```python
from build123d import *

# Parameters (mm, degrees)
TD_SKETCH_R                             = 0.79248
TL_FEATURE_DEPTH                        = 21.0312
TDF_STD_SKETCH_W                        = 2.09296
TDF_STD_SKETCH_H                        = 2.09296
TDF_STD_FEATURE_DEPTH                   = 22.061040395
ISA_20_STD_FEATURE_DEPTH                = 22.061040395
ISA_20_STD_FEATURE_DEPTH_BACK           = 22.061040395
VW_STD_FEATURE_DEPTH                    = 22.061040395
VW_STD_FEATURE_DEPTH_BACK               = 22.061040395
F_10BA_STD_FEATURE_DEPTH                = 22.061040503
F_10BA_STD_FEATURE_DEPTH_BACK           = 22.061040503
FRO_STD_FEATURE_DEPTH                   = 22.061040395
FRO_STD_FEATURE_DEPTH_BACK              = 22.061040395
C_STD_FEATURE_DEPTH                     = 22.061040395
C_STD_FEATURE_DEPTH_BACK                = 22.061040395
ERW_STD_FEATURE_DEPTH                   = 0.018159984
H_STD_FEATURE_REACH                     = 22.957
H_STD_SKETCH_R                          = 0.01778
H_STD_SKETCH_3_R                        = 0.01778
FUNNEL_FINAL_DIAMETRE_STD_FEATURE_DEPTH = 2.499995
FUNNEL_FINAL_DIAMETRE_STD_FEATURE_DRAFT = -22.5
ROUND_BR_STD_FEATURE_START              = -1
ROUND_BR_STD_FEATURE_DEPTH              = 0.936596355


with BuildPart() as part:
    # TD_sketch → TL_feature (new body)
    with BuildSketch(Plane(origin=(0, 0, 0), x_dir=(1, 0, 0), z_dir=(0, 1, 0))):
        with Locations(Location((0, 0, 0), (0, 0, 270))):
            Circle(TD_SKETCH_R)
    extrude(amount=TL_FEATURE_DEPTH)

    # TDF_STD_sketch → TDF_STD_feature (cut, through all)
    with BuildSketch(Plane(origin=(0, 0, 0), x_dir=(1, 0, 0), z_dir=(0, 1, 0))):
        with Locations((-1.4224, 0)):
            Rectangle(TDF_STD_SKETCH_W, TDF_STD_SKETCH_H)
    extrude(amount=TDF_STD_FEATURE_DEPTH, mode=Mode.SUBTRACT)

    # ISA_20_STD_sketch → ISA_20_STD_feature (cut, two sides: drawn at the far end of the back side and taken through both)
    with BuildSketch(Plane(origin=(0, 0, 0), x_dir=(0, 0, -1), z_dir=(1, 0, 0)).offset(-ISA_20_STD_FEATURE_DEPTH_BACK)):
        Polygon((-12.948362797, 73.253751326), (-3.740117997, 21.0312), (-0.03175, 0), (0.03175, 0), (3.740117997, 21.0312), (12.948362797, 73.253751326), (12.948362797, -32.802585388), (-12.948362797, -32.802585388), align=None)
    extrude(amount=ISA_20_STD_FEATURE_DEPTH + ISA_20_STD_FEATURE_DEPTH_BACK, mode=Mode.SUBTRACT)

    # VW_STD_sketch → VW_STD_feature (cut, two sides: drawn at the far end of the back side and taken through both)
    with BuildSketch(Plane(origin=(0, 0, 0), x_dir=(0, 0, -1), z_dir=(1, 0, 0)).offset(-VW_STD_FEATURE_DEPTH_BACK)):
        with BuildLine():
            Line((-70.567982417, 70.76464549), (-20.834536927, 21.0312))
            Line((-20.834536927, 21.0312), (-0.060418463, 0.257081537))
            ThreePointArc((-0.060418463, 0.257081537), (-0.04390038, 0.232360478), (-0.0381, 0.2032))
            Line((-0.0381, 0.2032), (-0.0381, 0))
            Line((-0.0381, 0), (0.0381, 0))
            Line((0.0381, 0), (0.0381, 0.2032))
            ThreePointArc((0.0381, 0.2032), (0.04390038, 0.232360478), (0.060418463, 0.257081537))
            Line((0.060418463, 0.257081537), (20.834536927, 21.0312))
            Line((20.834536927, 21.0312), (70.567982417, 70.76464549))
            Line((70.567982417, 70.76464549), (70.567982417, -69.902780741))
            Line((70.567982417, -69.902780741), (-70.567982417, -69.902780741))
            Line((-70.567982417, -69.902780741), (-70.567982417, 70.76464549))
        make_face()
    extrude(amount=VW_STD_FEATURE_DEPTH + VW_STD_FEATURE_DEPTH_BACK, mode=Mode.SUBTRACT)

    # 10BA_STD_sketch → 10BA_STD_feature (cut, two sides: drawn at the far end of the back side and taken through both)
    with BuildSketch(Plane.XY.offset(-F_10BA_STD_FEATURE_DEPTH_BACK)):
        Polygon((-53.187772193, 0), (-0.37592, 0), (-0.2921, 0), (-0.091550146, 0.028185444), (3.611847997, 21.0312), (12.782529889, 73.04072149), (91.167207648, 2.243763782), (25.196905566, -70.796957708), align=None)
    extrude(amount=F_10BA_STD_FEATURE_DEPTH + F_10BA_STD_FEATURE_DEPTH_BACK, mode=Mode.SUBTRACT)

    # FRO_STD_sketch → FRO_STD_feature (cut, two sides: drawn at the far end of the back side and taken through both)
    with BuildSketch(Plane.XY.offset(-FRO_STD_FEATURE_DEPTH_BACK)):
        with BuildLine():
            Line((-0.37592, 52.152138388), (-0.37592, 0.02794))
            ThreePointArc((-0.37592, 0.02794), (-0.367736563, 0.008183437), (-0.34798, 0))
            Line((-0.34798, 0), (51.776218388, 0))
            Line((51.776218388, 0), (-21.9385299, -73.714748288))
            Line((-21.9385299, -73.714748288), (-74.090668288, -21.5626099))
            Line((-74.090668288, -21.5626099), (-0.37592, 52.152138388))
        make_face()
    extrude(amount=FRO_STD_FEATURE_DEPTH + FRO_STD_FEATURE_DEPTH_BACK, mode=Mode.SUBTRACT)

    # C_STD_sketch → C_STD_feature (cut, two sides: drawn at the far end of the back side and taken through both)
    with BuildSketch(Plane(origin=(0, 0, 0), x_dir=(0, 0, -1), z_dir=(1, 0, 0)).offset(-C_STD_FEATURE_DEPTH_BACK)):
        with BuildLine():
            Line((-50.530423385, -12.791040855), (-0.030559272, 0))
            ThreePointArc((-0.030559272, 0), (0, 0.00381), (0.030559272, 0))
            Line((0.030559272, 0), (50.530423385, -12.791040855))
            Line((50.530423385, -12.791040855), (50.530423385, -116.980234183))
            Line((50.530423385, -116.980234183), (-50.530423385, -116.980234183))
            Line((-50.530423385, -116.980234183), (-50.530423385, -12.791040855))
        make_face()
    extrude(amount=C_STD_FEATURE_DEPTH + C_STD_FEATURE_DEPTH_BACK, mode=Mode.SUBTRACT)


with BuildPart() as body_2:
    # ERW_STD_sketch → ERW_STD_feature (new, symmetric)
    with BuildSketch(Plane.XY):
        Polygon((-0.18288, 0.05842), (-0.18288, 0), (-0.32766, 0), (-0.283637372, 0.05842), align=None)
    extrude(amount=ERW_STD_FEATURE_DEPTH, both=True)

    # H_STD_sketch → H_STD_feature (add, up to next)
    with BuildSketch(Plane(origin=(-0.096399563, 0.108349503, 0), x_dir=(0, 0, -1), z_dir=(0.8660254037844415, 0.4999999999999953, 0)), mode=Mode.PRIVATE) as h_std_feature_sk1:
        with Locations(Location((0, 0, 0), (0, 0, 90))):
            Circle(H_STD_SKETCH_R)
    h_std_feature_tool1 = extrude(h_std_feature_sk1.sketch, amount=-H_STD_FEATURE_REACH, mode=Mode.PRIVATE) - body_2.part
    add(h_std_feature_tool1.solids().sort_by_distance((-0.0964, 0.10835, 0))[0])


with BuildPart() as funnel_final_diametre_std_feature_tool:
    # H_STD_sketch<3> → funnel_final_diametre_STD_feature (with draft: the straight prism first)
    with BuildSketch(Plane(origin=(-0.096399563, 0.108349503, 0), x_dir=(0, 0, -1), z_dir=(0.8660254037844415, 0.4999999999999953, 0))):
        with Locations(Location((0, 0, 0), (0, 0, 90))):
            Circle(H_STD_SKETCH_3_R)
    extrude(amount=FUNNEL_FINAL_DIAMETRE_STD_FEATURE_DEPTH)
    # funnel_final_diametre_STD_feature: the draft: its side faces are tilted about the plane it starts from
    funnel_final_diametre_std_feature_sides = [funnel_final_diametre_std_feature_tool.faces().sort_by_distance(p)[0] for p in [
        (0.995020026, 0.717950322, 0),
    ]]
    draft(funnel_final_diametre_std_feature_sides, Plane(origin=(-0.096399563, 0.108349503, 0), x_dir=(0, 0, -1), z_dir=(0.8660254037844415, 0.4999999999999953, 0)), FUNNEL_FINAL_DIAMETRE_STD_FEATURE_DRAFT)


with BuildPart() as body_2_1:
    add(body_2.part)

    # funnel_final_diametre_STD_feature: add funnel_final_diametre_std_feature_tool
    add(funnel_final_diametre_std_feature_tool.part)

    # ROUND_BR_STD_feature: read off the stored shape, not the designer's step
    # ROUND_BR_STD_feature outline → ROUND_BR_STD_feature (cut)
    with BuildSketch(Plane(origin=(0, 0, 0), x_dir=(0.79863551004729, -0.601815023152052, 0), z_dir=(0.601815023152052, 0.79863551004729, 0)).offset(ROUND_BR_STD_FEATURE_START)):
        with BuildLine():
            Line((-0.261680911, -0.018159984), (-0.243520927, -0.018159984))
            ThreePointArc((-0.243520927, -0.018159984), (-0.256361975, -0.012841048), (-0.261680911, 0))
            Line((-0.261680911, 0), (-0.261680911, -0.018159984))
        make_face()
        with BuildLine():
            Line((-0.261680911, 0.018159984), (-0.261680911, 0))
            ThreePointArc((-0.261680911, 0), (-0.256361975, 0.012841048), (-0.243520927, 0.018159984))
            Line((-0.243520927, 0.018159984), (-0.261680911, 0.018159984))
        make_face()
    extrude(amount=ROUND_BR_STD_FEATURE_DEPTH, mode=Mode.SUBTRACT)


with BuildPart() as part_1:
    add(part.part)

    # COMBINE_STD_feature: cut body 2
    add(body_2_1.part, mode=Mode.SUBTRACT)


solid = part_1.part
```
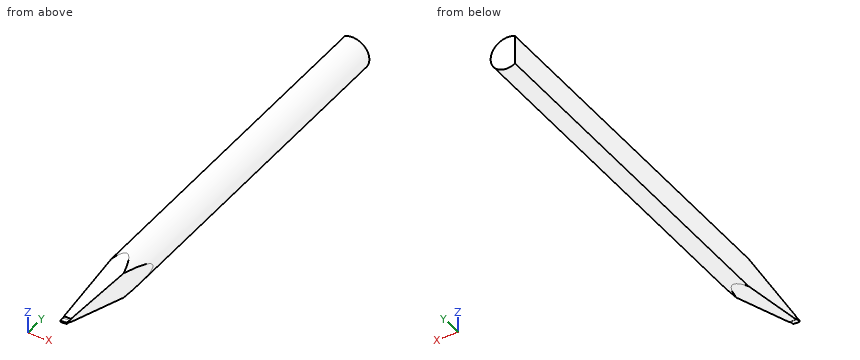
Geometry: final body of the model. Coordinates: model frame, mm. Round coordinates to 2 decimals unless told otherwise and drop trailing zeros. Write each loop counter-clockwise with the first axis right and the second up, starting at its lowest first coordinate (ties: lowest second). Pieces come first, ordered by that corner, then holes.
Item 1: Section query B-B (z = 0.4). Return loops of the section in (x, y), plus the area to 3 significant figures.
Item 2: Material intervals for L1, parallel to X at y = 9.75, z = -0.05; L2, parallel to Z at x = 0.05, y = 16.75; L3, parallel to X at y = 14.75, z = -0.65, sorted ascending.
Item 3: Section query A-A (y = 18.25). Return loops of the section in (x, z).
Item 4: Section query C-C (x = 0.15). Return loops of the section in (y, z).
Completed:
1. outline: (-0.38, 2.09) - (0.27, 2.09) - (0.68, 4.43) - (0.68, 21.03) - (-0.38, 21.03) - close
1. area: 19.6 mm2
2. L1: x = -0.38 to 0.79
2. L2: z = -0.79 to 0.79
2. L3: x = -0.38 to 0.45
3. outline: (-0.38, -0.7) arc R0.79 ccw (long way) to (-0.38, 0.7) - close
4. outline: (1.4, -0.28) - (4.23, -0.78) - (21.03, -0.78) - (21.03, 0.78) - (4.23, 0.78) - (1.4, 0.28) - close
